Input: part model. Units: mm. Frame: model coordinates. Face numbers are marked on the shaded views. A direction names the side the tool comes from. Round coordinates to 2 decimals unless told otherwise and drop trailing zeros. Order: outer loops, then holes, each group sorted by start corner. A loop starts at its lowest first (then second) coordinate and runs counter-clockwise, first axis right, second up. Notation, with made-up numbers: (67, 53) - (89, 53) arc R25 ccw to (89, 91) - close; hole circle Ø11 at (44.25, 38.25). An arc over 180 degrees is marked (long way). One line per item, written item: value. Start each with the question number.
from build123d import *

# Parameters (mm, degrees)
SKETCH1_W           = 420
SKETCH1_H           = 420
SKETCH1_R           = 33.203133877
BOSS_EXTRUDE2_DEPTH = 250
BOSS_EXTRUDE3_DEPTH = 1
SKETCH4_RX          = 216.159218744
SKETCH4_RY          = 124.438636569
BOSS_EXTRUDE4_DEPTH = 31
SKETCH5_RX          = 136.808799133
SKETCH5_RY          = 69.0562156
BOSS_EXTRUDE5_DEPTH = 51


with BuildPart() as part:
    # Sketch1 → Boss-Extrude2 (new body)
    with BuildSketch(Plane.XY):
        with Locations((-1046.276969261, 563.504412843)):
            Rectangle(SKETCH1_W, SKETCH1_H)
        with Locations((-986.276969261, 705.792386227)):
            Circle(SKETCH1_R, mode=Mode.SUBTRACT)
        with Locations((-1106.276969261, 705.792386227)):
            Circle(SKETCH1_R, mode=Mode.SUBTRACT)
        Polygon((-1026.007137098, 619.07974314), (-1045.889944458, 649.563457617), (-1062.401956466, 619.07974314), align=None, mode=Mode.SUBTRACT)
        with BuildLine():
            Line((-1144.96201651, 469.201480292), (-925.225241317, 469.201480292))
            add(Edge.make_bspline(
                [(-1144.96201651, 469.201480292), (-1132.834759851, 516.055423689), (-1038.44686365, 538.622906956), (-948.523344563, 517.634809157), (-925.225241317, 469.201480292)],
                knots=[0, 0, 0, 0, 0.465700798, 1, 1, 1, 1], degree=3))
        make_face(mode=Mode.SUBTRACT)
    extrude(amount=BOSS_EXTRUDE2_DEPTH)

    # Sketch2 → Boss-Extrude3 (add)
    with BuildSketch(Plane.XY.offset(250)):
        with BuildLine():
            Line((-1122.462851099, 659.218542915), (-1128.539059101, 640.437536361))
            ThreePointArc((-1128.539059101, 640.437536361), (-1128.529323469, 639.793287222), (-1128.128635759, 639.288707105))
            add(Edge.make_bspline(
                [(-1128.128635759, 639.288707105), (-1127.290338361, 638.749430284), (-1125.582255263, 638.18298139), (-1123.857803216, 638.640795026), (-1122.979860291, 639.125064157)],
                knots=[0.103294074, 0.103294074, 0.103294074, 0.103294074, 0.51185707, 0.920052959, 0.920052959, 0.920052959, 0.920052959], degree=3))
            ThreePointArc((-1122.979860291, 639.125064157), (-1122.601749825, 639.492256106), (-1122.462851099, 640.000689579))
            Line((-1122.462851099, 640.000689579), (-1122.462851099, 659.218542915))
        make_face()
    extrude(amount=BOSS_EXTRUDE3_DEPTH)

    # Sketch4 → Boss-Extrude4 (add)
    with BuildSketch(Plane(origin=(0, 773.504412843, 0), x_dir=(1, 0, 0), z_dir=(0, 1, 0))):
        with Locations(Location((-1047.356098163, -122.204602032), (0, 0, 167.772053481))):
            Ellipse(SKETCH4_RX, SKETCH4_RY)
    extrude(amount=BOSS_EXTRUDE4_DEPTH)

    # Sketch5 → Boss-Extrude5 (add)
    with BuildSketch(Plane(origin=(0, 804.504412843, 0), x_dir=(1, 0, 0), z_dir=(0, 1, 0))):
        with Locations(Location((-1044.407129707, -130.546272111), (0, 0, -14.547039262))):
            Ellipse(SKETCH5_RX, SKETCH5_RY)
    extrude(amount=BOSS_EXTRUDE5_DEPTH)


solid = part.part
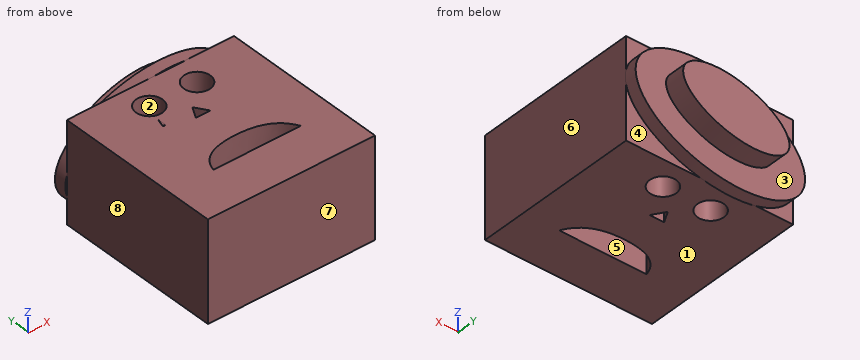
Item 1: Reachability of the marked faces 1, 2, 3 and 4 from +Z, -Z, +X, -X, +Y, -Y: full face, straight path, thin tool, end or side. Return the list, or none.
Item 2: First-contact query: pin 1 Ø2 at (y, z) = (609, 203) entering from +X; pin 2 Ø10 at (x, y) = (-1158, 448.5) entering from +Z; pin 3 Ø12 at (x, y) = (-1165.5, 489) entering from -Z. Flat tips, straight axial feed; report the tip coordinate or a pass-through.
Item 3: Section query A-A on y = 694. Return loops of the section in (x, z).
Item 4: Pull-direction query (X, two-part tool) for the marked faces 5, 6, 7 and 8; classes: released by +X, released by -X, zero draft, split by the parting line, or undercut.
Item 5: Section query B-B on x = -993.5. Give the number of separate pieces and of enclosed holes in the cut face, and give its area (3 significant figures).
Item 6: Section query D-D on y = 429. Return loops of the section in (x, z).
Item 7: Line query: L1, parallel to X at y = 685, z = 167.5; L2, parallel to Y at x = -1005, z = 103; L3, parallel to Y at x = -1010.5, z = 175. Output: solid intervals per line, ascending.
Geometry results:
1. face 1: -Z, +X, -X, -Y
1. face 2: +Z, -Z
1. face 3: +Y
1. face 4: -Z, +X, +Y
2. pin 1: stops at x = -836.28
2. pin 2: stops at z = 250
2. pin 3: stops at z = 0
3. outline: (-1256.28, 0) - (-1137.32, 0) - (-1137.32, 250) - (-1256.28, 250) - close; (-1075.24, 0) - (-1017.32, 0) - (-1017.32, 250) - (-1075.24, 250) - close; (-955.24, 0) - (-836.28, 0) - (-836.28, 250) - (-955.24, 250) - close
4. face 5: undercut
4. face 6: released by +X
4. face 7: zero draft
4. face 8: released by -X
5. separate pieces: 3
5. enclosed holes: 0
5. area: 89,700 mm^2
6. outline: (-1256.28, 0) - (-836.28, 0) - (-836.28, 250) - (-1256.28, 250) - close
7. L1: x = -1256.28 to -1132.16, -1080.39 to -1012.16, -960.39 to -836.28
7. L2: y = 353.5 to 469.2, 525.14 to 678.37, 733.21 to 855.5
7. L3: y = 353.5 to 469.2, 525.96 to 683.08, 728.5 to 855.5
